from build123d import *

# Parameters (mm, degrees)
SKETCH1_R                = 2.1
BOSS_EXTRUDE1_DEPTH      = 2.54
BOSS_EXTRUDE2_DEPTH      = 25.4
BOSS_EXTRUDE2_DEPTH_BACK = 2.54
SKETCH2_W                = 45.847007751
SKETCH2_H                = 2.54
FILLET1_R                = 2


with BuildPart() as part:
    # Sketch1 → Boss-Extrude1 (new body)
    with BuildSketch(Plane(origin=(0, 0, 0), x_dir=(1, 0, 0), z_dir=(0, 1, 0))):
        Polygon((15.569104138, 29.110597295), (25.03510725, 29.110597295), (25.03510725, 3.075596379), (51.56910725, 3.075596379), (51.56910725, 29.110597295), (61.416111889, 29.110597295), (61.416111889, -2.131403285), (61.416111889, -3.401403285), (15.569104138, -3.401403285), (15.569104138, -2.131403285), align=None)
        with Locations(Location((20.39510725, 23.395596379, 0), (0, 0, 270))):
            Circle(SKETCH1_R, mode=Mode.SUBTRACT)
        with Locations(Location((20.39510725, 3.075596379, 0), (0, 0, 270))):
            Circle(SKETCH1_R, mode=Mode.SUBTRACT)
        with Locations(Location((56.20910725, 23.395596379, 0), (0, 0, 270))):
            Circle(SKETCH1_R, mode=Mode.SUBTRACT)
        with Locations(Location((56.20910725, 3.075596379, 0), (0, 0, 270))):
            Circle(SKETCH1_R, mode=Mode.SUBTRACT)
    extrude(amount=BOSS_EXTRUDE1_DEPTH)

    # Sketch2 → Boss-Extrude2 (add, two sides: drawn at the far end of the back side and taken through both)
    with BuildSketch(Plane.XZ.offset(-BOSS_EXTRUDE2_DEPTH_BACK)):
        with Locations((38.492608014, 4.671403285)):
            Rectangle(SKETCH2_W, SKETCH2_H)
    extrude(amount=BOSS_EXTRUDE2_DEPTH + BOSS_EXTRUDE2_DEPTH_BACK)

    # Fillet1
    fillet1_edges = [part.edges().sort_by_distance(p)[0] for p in [
        (38.492608013, 0, 3.401403285),
        (15.569104138, 1.27, -29.110597295),
        (25.03510725, 1.27, -29.110597295),
        (25.03510725, 1.27, -3.075596379),
        (51.56910725, 1.27, -3.075596379),
        (51.56910725, 1.27, -29.110597295),
        (61.416111889, 1.27, -29.110597295),
        (15.569104138, -25.4, 4.671403285),
        (61.416111889, -25.4, 4.671403285),
    ]]
    fillet(fillet1_edges, radius=FILLET1_R)


solid = part.part
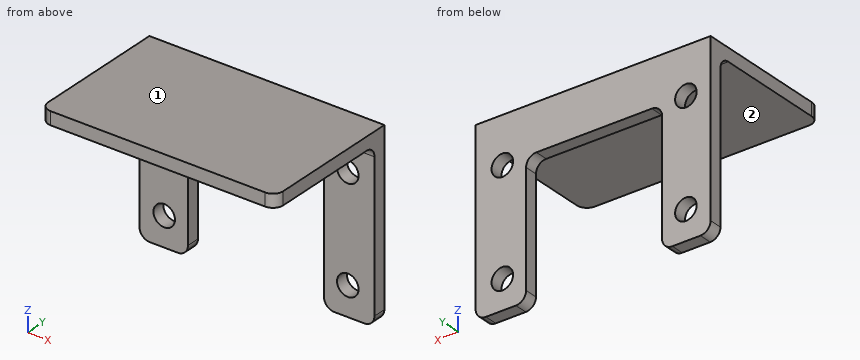
The model under review builds one solid part; all positions refer to its coordinate system, in mm. Face numbers are marked on the shaded views. A direction names the side the tool comes from. Coordinates: 2 decimals unless noted, no trailing zeros. Loops run counter-clockwise (first coordinate to the right, second up) from the corner with the lowest first, then second, coordinate; pieces in that order, holes last.
(1) Wall thickness on L1, parallel to Z at x = 33.5, y = -5; L2, parallel to X at y = 0.5, z = -25; L3, parallel to Y at x = 21, z = -18: over which ranges is each line inside the solid? List them lowest first.
Determined:
L1: z = 3.4 to 5.94
L2: x = 15.57 to 19.04, 21.75 to 25.04, 51.57 to 54.85, 57.56 to 61.42
L3: y = 0 to 2.54
(2) Consider section A-A, the plane z = -20. Give the boundary of the cut face in (x, y), plus the area to 3 significant figures.
Determined:
outline: (15.57, 0) - (25.04, 0) - (25.04, 2.54) - (15.57, 2.54) - close; (51.57, 0) - (61.42, 0) - (61.42, 2.54) - (51.57, 2.54) - close
area: 49.1 mm2
(3) Consider section C-C, the plane y = -7. Give the boundary of the cut face in (x, z), plus the area to 3 significant figures.
Determined:
outline: (15.57, 3.4) - (61.42, 3.4) - (61.42, 5.94) - (15.57, 5.94) - close
area: 116 mm2
(4) Consider section B-B, the plane x = 40. Give the boundary of the cut face in (y, z).
Determined:
outline: (-25.4, 3.4) - (-2, 3.4) arc R2 cw to (0, 1.4) - (0, -3.08) - (2.54, -3.08) - (2.54, 5.94) - (-25.4, 5.94) - close
(5) Tool access review of the marked faces 1 and 2: name each direction out of +Z, -Z, +X, -X, +Y, -Y from which nothing blocks a thin tool from reaching the whole face with its end or side.
Determined:
face 1: +Z, +X, -X, +Y, -Y
face 2: -Z, +X, -X, -Y
(6) Insertion check: P1, Ø6.5, axis at x = 20.4, z = -3.08, coming from the -Y side; P2, Ø1.3, axis at x = 37, y = 0.5, coming from the -Z side. Each pin has a flat end and moves straight along its axis. Give the tip position at first contact, or say it passes through.
Determined:
P1: stops at y = 0
P2: stops at z = -3.08
